```python
from build123d import *

# Parameters (mm, degrees)
F0_R          = 3
F0_R_2        = 2.5
F1_DEPTH      = 282
F2_R          = 2
F3_R          = 7
F6_DEPTH      = 30
F6_DEPTH_BACK = 30


# Not quite as in the source:
# - a feature names something its author has since deleted; it is built from what else it names


with BuildPart() as f1:
    # F0 (on Top) → F1 (new body)
    with BuildSketch(Plane.XY):
        with BuildLine():
            Line((18.15, -30), (30, -30))
            Line((30, -30), (30, -18.15))
            Line((30, -18.15), (27.5, -18.15))
            Line((27.5, -18.15), (27.5, -20.15))
            Line((27.5, -20.15), (21.5477069044, -20.15))
            ThreePointArc((21.5477069044, -20.15), (19.5, -15), (21.5477069044, -9.85))
            Line((21.5477069044, -9.85), (27.5, -9.85))
            Line((27.5, -9.85), (27.5, -11.85))
            Line((27.5, -11.85), (30, -11.85))
            Line((30, -11.85), (30, 11.85))
            Line((30, 11.85), (27.5, 11.85))
            Line((27.5, 11.85), (27.5, 9.85))
            Line((27.5, 9.85), (21.5477069044, 9.85))
            ThreePointArc((21.5477069044, 9.85), (19.5, 15), (21.5477069044, 20.15))
            Line((21.5477069044, 20.15), (27.5, 20.15))
            Line((27.5, 20.15), (27.5, 18.15))
            Line((27.5, 18.15), (30, 18.15))
            Line((30, 18.15), (30, 30))
            Line((30, 30), (18.15, 30))
            Line((18.15, 30), (18.15, 27.5))
            Line((18.15, 27.5), (20.15, 27.5))
            Line((20.15, 27.5), (20.15, 21.5477069044))
            ThreePointArc((20.15, 21.5477069044), (15, 19.5), (9.85, 21.5477069044))
            Line((9.85, 21.5477069044), (9.85, 27.5))
            Line((9.85, 27.5), (11.85, 27.5))
            Line((11.85, 27.5), (11.85, 30))
            Line((11.85, 30), (-11.85, 30))
            Line((-11.85, 30), (-11.85, 27.5))
            Line((-11.85, 27.5), (-9.85, 27.5))
            Line((-9.85, 27.5), (-9.85, 21.5477069044))
            ThreePointArc((-9.85, 21.5477069044), (-15, 19.5), (-20.15, 21.5477069044))
            Line((-20.15, 21.5477069044), (-20.15, 27.5))
            Line((-20.15, 27.5), (-18.15, 27.5))
            Line((-18.15, 27.5), (-18.15, 30))
            Line((-18.15, 30), (-30, 30))
            Line((-30, 30), (-30, 18.15))
            Line((-30, 18.15), (-27.5, 18.15))
            Line((-27.5, 18.15), (-27.5, 20.15))
            Line((-27.5, 20.15), (-21.5477069044, 20.15))
            ThreePointArc((-21.5477069044, 20.15), (-19.5, 15), (-21.5477069044, 9.85))
            Line((-21.5477069044, 9.85), (-27.5, 9.85))
            Line((-27.5, 9.85), (-27.5, 11.85))
            Line((-27.5, 11.85), (-30, 11.85))
            Line((-30, 11.85), (-30, -11.85))
            Line((-30, -11.85), (-27.5, -11.85))
            Line((-27.5, -11.85), (-27.5, -9.85))
            Line((-27.5, -9.85), (-21.5477069044, -9.85))
            ThreePointArc((-21.5477069044, -9.85), (-19.5, -15), (-21.5477069044, -20.15))
            Line((-21.5477069044, -20.15), (-27.5, -20.15))
            Line((-27.5, -20.15), (-27.5, -18.15))
            Line((-27.5, -18.15), (-30, -18.15))
            Line((-30, -18.15), (-30, -30))
            Line((-30, -30), (-18.15, -30))
            Line((-18.15, -30), (-18.15, -27.5))
            Line((-18.15, -27.5), (-20.15, -27.5))
            Line((-20.15, -27.5), (-20.15, -21.5477069044))
            ThreePointArc((-20.15, -21.5477069044), (-15, -19.5), (-9.85, -21.5477069044))
            Line((-9.85, -21.5477069044), (-9.85, -27.5))
            Line((-9.85, -27.5), (-11.85, -27.5))
            Line((-11.85, -27.5), (-11.85, -30))
            Line((-11.85, -30), (11.85, -30))
            Line((11.85, -30), (11.85, -27.5))
            Line((11.85, -27.5), (9.85, -27.5))
            Line((9.85, -27.5), (9.85, -21.5477069044))
            ThreePointArc((9.85, -21.5477069044), (15, -19.5), (20.15, -21.5477069044))
            Line((20.15, -21.5477069044), (20.15, -27.5))
            Line((20.15, -27.5), (18.15, -27.5))
            Line((18.15, -27.5), (18.15, -30))
        make_face()
        with Locations((-25, -25)):
            Circle(F0_R, mode=Mode.SUBTRACT)
        with Locations((-15, -15)):
            Circle(F0_R_2, mode=Mode.SUBTRACT)
        with Locations((25, -25)):
            Circle(F0_R, mode=Mode.SUBTRACT)
        with Locations((15, -15)):
            Circle(F0_R_2, mode=Mode.SUBTRACT)
        with Locations((-25, 25)):
            Circle(F0_R, mode=Mode.SUBTRACT)
        with Locations((-15, 15)):
            Circle(F0_R_2, mode=Mode.SUBTRACT)
        Polygon((-7, 22), (-7, 27.5), (0, 27.5), (7, 27.5), (7, 22), (10, 16), (10, 10), (16, 10), (22, 7), (27.5, 7), (27.5, 0), (27.5, -7), (22, -7), (16, -10), (10, -10), (10, -16), (7, -22), (7, -27.5), (0, -27.5), (-7, -27.5), (-7, -22), (-10, -16), (-10, -10), (-16, -10), (-22, -7), (-27.5, -7), (-27.5, 0), (-27.5, 7), (-22, 7), (-16, 10), (-10, 10), (-10, 16), align=None, mode=Mode.SUBTRACT)
        with Locations((15, 15)):
            Circle(F0_R_2, mode=Mode.SUBTRACT)
        with Locations((25, 25)):
            Circle(F0_R, mode=Mode.SUBTRACT)
    extrude(amount=F1_DEPTH)

    # F2
    f2_edges = [f1.edges().sort_by_distance(p)[0] for p in [
        (-7, 27.5, 141),
        (7, 27.5, 141),
    ]]
    fillet(f2_edges, radius=F2_R)

    # F3
    f3_edges = [f1.edges().sort_by_distance(p)[0] for p in [
        (-10, 16, 141),
        (10, 16, 141),
    ]]
    fillet(f3_edges, radius=F3_R)

    # F5 (on Right) → F6 (cut, two sides)
    with BuildSketch(Plane.YZ) as f6_sk:
        Polygon((115.2614038106, 44.5196963257), (64.8905500682, 94.8905500682), (-30, 0), (20.3708537424, -50.3708537424), align=None)
        Polygon((30, 282), (-7.7241411908, 373.0741332917), (-157.9632044753, 310.843075681), (-120.2390632845, 219.7689423893), align=None)
    extrude(amount=F6_DEPTH, mode=Mode.SUBTRACT)
    extrude(f6_sk.sketch, amount=-F6_DEPTH_BACK, mode=Mode.SUBTRACT)


solid = f1.part
```
Geometry check sheet. Reference: the model listing, model coordinates, mm. Coordinates: 2 decimals unless noted, no trailing zeros. Order: outer loops, then holes, each group sorted by start corner. A loop starts at its lowest first (then second) coordinate and runs counter-clockwise, first axis right, second up.
Item 1: Section check A-A (y = -25). Enter the section's corners in (x, z).
Item 2: Section check B-B (y = -4.5). Enter the section's corners in (x, z), plus the area to 3 significant figures.
Item 3: Depth check by flat-ended pin: pin 1 (3.5 mm diameter, centred on x = 25, y = 25, fed in from -Z); pin 2 (8 mm diameter, centred on x = 15, y = 15, fed in from +Z); pin 3 (1.3 mm diameter, centred on y = 13, z = 213.5, fed in from +X); pin 4 (1.8 mm diameter, centred on x = 14, z = 195.5, fed in from -Y). Enter the tip coordinate at first touch or a pass-through.
Item 4: Scan lines: line 1 along Y through (x, z) = (15, 170); line 2 along X through (y, z) = (-25, 161). Record each from-to range of solid material in increasing order.
Item 5: Mould release check, pull along X, two halves, no side actions. Record for faces 1 (the cylindrical face through (12.5, -14.9, 136.7)), 2 (the flat face through (-30, -24, 129)), 3 (the flat face through (-25, -7, 143)), 4 (the flat face through (24, -30, 127)): released by +X, released by -X, zero draft, split by the parting line, or undercut.
Item 6: Section check C-C (z = 193). Count the separate pieces of the cut face and the enclosed holes in it, plus the area to 3 significant figures.
Check sheet entries:
1. outline: (-30, 5) - (-28, 5) - (-28, 259.22) - (-30, 259.22) - close; (-22, 5) - (-20.15, 5) - (-20.15, 259.22) - (-22, 259.22) - close; (-9.85, 5) - (-7, 5) - (-7, 259.22) - (-9.85, 259.22) - close; (7, 5) - (9.85, 5) - (9.85, 259.22) - (7, 259.22) - close; (20.15, 5) - (22, 5) - (22, 259.22) - (20.15, 259.22) - close; (28, 5) - (30, 5) - (30, 259.22) - (28, 259.22) - close
2. outline: (-30, 25.5) - (-27.5, 25.5) - (-27.5, 267.71) - (-30, 267.71) - close; (27.5, 25.5) - (30, 25.5) - (30, 267.71) - (27.5, 267.71) - close
2. area: 1,210 mm2
3. pin 1: passes through
3. pin 2: stops at z = 277.44
3. pin 3: stops at x = 19.98
3. pin 4: stops at y = -19.74
4. line 1: y = -19.5 to -17.5, -12.5 to -10, 10 to 12.5, 17.5 to 19.5
4. line 2: x = -30 to -28, -22 to -20.15, -9.85 to -7, 7 to 9.85, 20.15 to 22, 28 to 30
5. face 1: undercut
5. face 2: released by -X
5. face 3: undercut
5. face 4: zero draft
6. separate pieces: 1
6. enclosed holes: 9
6. area: 1,080 mm2
